Autodesk Inventor part; units mm, degrees
ref_plane "YZ Plane" through (0, 0, 0) normal (1, 0, 0) x (0, 1, 0)
ref_plane "XZ Plane" through (0, 0, 0) normal (0, 1, 0) x (-1, 0, 0)
ref_plane "XY Plane" through (0, 0, 0) normal (0, 0, 1) x (1, 0, 0)
sketch "Block1" plane through (0, 0, 0) normal (0, 0, 1) x (1, 0, 0)
  circle A0 centre (0, 0) radius 50.22
  circle A1 centre (-30, -32.5) radius 2.72
  circle A2 centre (30, -32.5) radius 2.72
  circle A3 centre (0, 0) radius 5.22
  circle A4 centre (-30, 32.5) radius 2.72
  circle A5 centre (30, 32.5) radius 2.72
sketch "Block2" plane through (0, 0, 0) normal (0, 0, 1) x (1, 0, 0)
  circle A0 centre (0, 0) radius 35.22
  circle A1 centre (0, 0) radius 5.22
  circle A2 centre (20, 20) radius 2.72
  circle A3 centre (-20, 20) radius 2.72
  circle A4 centre (-20, -20) radius 2.72
  circle A5 centre (20, -20) radius 2.72
  point P0 (0, 0)
sketch "Block3" plane through (0, 0, 0) normal (0, 0, 1) x (1, 0, 0)
  circle A0 centre (0, 0) radius 35.22
  circle A1 centre (-15, 17.5) radius 2.72
  circle A2 centre (0, 0) radius 5.22
  circle A3 centre (-15, -17.5) radius 2.72
  circle A4 centre (15, 17.5) radius 2.72
  circle A5 centre (15, -17.5) radius 2.72
sketch "Block4" plane through (0, 0, 0) normal (0, 0, 1) x (1, 0, 0)
  circle A0 centre (0, 0) radius 35.22
  circle A1 centre (-15, 15) radius 2.72
  circle A2 centre (-15, -15) radius 2.72
  circle A3 centre (0, 0) radius 5.22
  circle A4 centre (15, 15) radius 2.72
  circle A5 centre (15, -15) radius 2.72
sketch "Sketch1" plane through (0, 0, 0) normal (0, 1, 0) x (-1, 0, 0)
  circle A0 centre (0, 0) radius 35
  line L0 (49, 0) -> (-49, 0)
  line L1 (0, -49) -> (0, 49)
  circle A1 centre (-15, -15) radius 2.5
  circle A2 centre (15, -15) radius 2.5
  circle A3 centre (-15, 15) radius 2.5
  circle A4 centre (15, 15) radius 2.5
  circle A5 centre (0, 0) radius 5
  dimension "d0" = 70
  dimension "d29" = 5
  dimension "d30" = 15
  dimension "d31" = 15
  dimension "d34" = 10
extrude "Extrusion5" add sketch "Sketch1" along normal blind 30 contours L0 A5 L1 A0 | A0 L1 A5 L0 | L1 A5 L0 A0 | A0 L0 A5 L1
sketch "Sketch9" plane through (0, 0, 0) normal (0, -1, 0) x (1, 0, 0)
  circle A0 centre (0, 0) radius 5
  circle A1 centre (-15, 15) radius 2.5
  circle A2 centre (15, 15) radius 2.5
  circle A3 centre (-15, -15) radius 2.5
  circle A4 centre (15, -15) radius 2.5
  circle A5 centre (0, 0) radius 35
sketch "DXF" plane through (0, 0, 0) normal (0, 1, 0) x (-1, 0, 0)
  point P0 (0, 0)
properties part number "drivepulleyMiddle"
The listing builds one solid part. Answer for the finished solid, in the listing's coordinates (mm). Coordinates: 2 decimals unless noted, no trailing zeros. Write each loop counter-clockwise with the first axis right and the second up, starting at its lowest first coordinate (ties: lowest second). Pieces come first, ordered by that corner, then holes. Notation, with made-up numbers: (-31.75, -9) - (4.25, -9) arc R20 ccw to (4.25, 1) - close; hole circle Ø9 at (27, -22). An arc over 180 degrees is marked (long way). Return JSON: item names as keys, results as strings. Group by question number.
Q1. Find the intervals of material crossed by line 1 along Z through (x, y) = (-15, 12); line 2 along X through (y, z) = (10.25, -14); line 3 along Z through (x, y) = (0, 13.5), in increasing order. Write a range as [from, to].
Q2. The part is cut by section C-C on z = 0. Write down the section's boundary in (x, y), and give its area (3 significant figures).
Q3. The part is cut by section B-B on x = 0. Write down the section's boundary in (y, z), and give its area (3 significant figures).
Q4. Flat-ended cylindrical pins translate along their axes: pin 1 Ø1 at (y, z) = (7, 27) entering from +X; pin 2 Ø10 at (y, z) = (14, -24) entering from +X; pin 3 Ø1.5 at (x, y) = (-27.5, 24.5) entering from -Z; pin 4 Ø4 at (x, z) = (15, -15) entering from +Y. Find the tip coordinate at first contact, or state that the pin passes through.
Q5. For a pull along Z with two mould halves and no side action, classify faces 1 (the cylindrical face through (-12.5, 14.8, -15.1)), 2 (the cylindrical face through (28, 15, 21)), 3 (the flat face through (0, 0, -7)), 4 (the cylindrical face through (17, 14.8, 16.5)) as +Z half, -Z half, draft (parallel to the pull), parting line (faces both ways), or undercut.
Q6. The part is cut by section D-D on x = 14.5. Write down the section's boundary in (y, z).
Q7. The part is cut by section A-A on z = -15. Write down the section's boundary in (x, y), and give its area (3 significant figures).
Evaluation:
{
 "1": {"line 1": "z = [-31.62, -17.5], [-12.5, 12.5], [17.5, 31.62]", "line 2": "x = [-32.08, -17.29], [-12.71, 12.71], [17.29, 32.08]", "line 3": "z = [-35, -5], [5, 35]"},
 "2": {"outline": "(-35, 0) - (-5, 0) - (-5, 30) - (-35, 30) - close; (5, 0) - (35, 0) - (35, 30) - (5, 30) - close", "area": "1,800 mm2"},
 "3": {"outline": "(0, -35) - (30, -35) - (30, -5) - (0, -5) - close; (0, 5) - (30, 5) - (30, 35) - (0, 35) - close", "area": "1,800 mm2"},
 "4": {"pin 1": "stops at x = 22.86", "pin 2": "stops at x = 29.39", "pin 3": "stops at z = -22.57", "pin 4": "passes through"},
 "5": {"face 1": "undercut", "face 2": "parting line", "face 3": "draft", "face 4": "undercut"},
 "6": {"outline": "(0, -31.86) - (30, -31.86) - (30, -17.45) - (0, -17.45) - close; (0, -12.55) - (30, -12.55) - (30, 12.55) - (0, 12.55) - close; (0, 17.45) - (30, 17.45) - (30, 31.86) - (0, 31.86) - close"},
 "7": {"outline": "(-31.62, 0) - (-17.5, 0) - (-17.5, 30) - (-31.62, 30) - close; (-12.5, 0) - (12.5, 0) - (12.5, 30) - (-12.5, 30) - close; (17.5, 0) - (31.62, 0) - (31.62, 30) - (17.5, 30) - close", "area": "1,600 mm2"}
}
